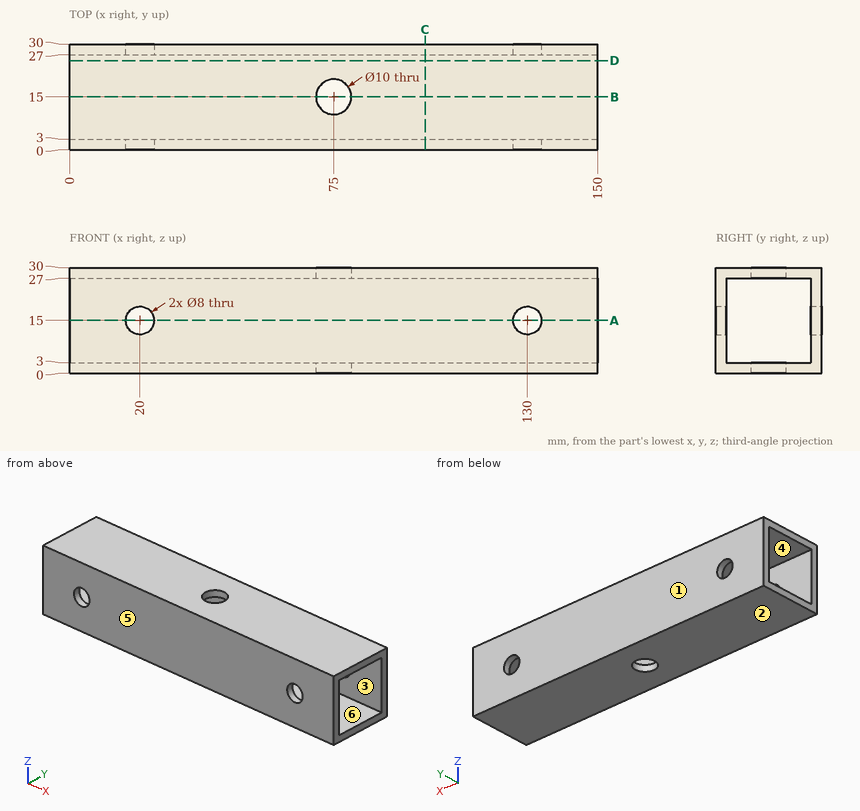
Part print with two shaded views. Sizes in mm from the minimum x, y, z corner. A direction names the side the tool comes from. Give positions to 0.01 mm unless a question says otherwise; leave off trailing zeros. Order: outer loops, then holes, each group sorted by start corner. A loop starts at its lowest first (then second) coordinate and runs counter-clockwise, first axis right, second up. Notation, with made-up numbers: M -34,57 L 20,57 A15 ccw 20,67 Z; hole C 79.5,2 d8. An arc over 180 degrees is marked long. Use one line per item in the form item = value.
1) Saw through at B-B (y = 15). Give the cut face in (x, z), plus the area to 3 significant figures.
Calculated:
outline = M 0,0 L 70,0 L 70,3 L 0,3 Z; M 0,27 L 70,27 L 70,30 L 0,30 Z; M 80,0 L 150,0 L 150,3 L 80,3 Z; M 80,27 L 150,27 L 150,30 L 80,30 Z
area = 840 mm2
2) Tool access for the marked faces 5 and 6: list every direction of +Z, -Z, +X, -X, +Y, -Y with a clear straight run to the whole face (end or side of a thin tool).
Calculated:
face_5 = +Z, -Z, +X, -X, -Y
face_6 = +X, -X
3) Saw through at C-C (x = 101). Give the cut face in (y, z), plus the area to 3 significant figures.
Calculated:
outline = M 0,0 L 30,0 L 30,30 L 0,30 Z; hole M 3,3 L 27,3 L 27,27 L 3,27 Z
area = 324 mm2
4) Saw through at A-A (z = 15). Give the cut face in (x, y), plus the area to 3 significant figures.
Calculated:
outline = M 0,0 L 16,0 L 16,3 L 0,3 Z; M 0,27 L 16,27 L 16,30 L 0,30 Z; M 24,0 L 126,0 L 126,3 L 24,3 Z; M 24,27 L 126,27 L 126,30 L 24,30 Z; M 134,0 L 150,0 L 150,3 L 134,3 Z; M 134,27 L 150,27 L 150,30 L 134,30 Z
area = 804 mm2
5) Saw through at D-D (y = 25.25). Give the cut face in (x, z), plus the area to 3 significant figures.
Calculated:
outline = M 0,0 L 150,0 L 150,3 L 0,3 Z; M 0,27 L 150,27 L 150,30 L 0,30 Z
area = 900 mm2
6) Drop a flat-ended pin along its axis: pin 1 (6.5 mm diameter, centred on x = 20, z = 15, fed in from +Y). Give the stop position or say it passes through.
Calculated:
pin_1 = through
7) Two-plate mould, pull along Z, no slides. Class the marked faces 1, 2, 3 and 4: released by +Z, released by -Z, zero draft, split by the parting line, or undercut.
Calculated:
face_1 = zero draft
face_2 = released by -Z
face_3 = undercut
face_4 = undercut
8) Probe probe 1 along X at (y, z) = (1.4, 15); probe 2 along Z at (x, y) = (121.5, 7). List the from-to ranges inside material, lowest first.
Calculated:
probe_1 = 0 to 16, 24 to 126, 134 to 150
probe_2 = 0 to 3, 27 to 30
